Input: part model. Units: mm. Frame: model coordinates. A direction names the side the tool comes from. Give positions to 0.01 mm unless a question says otherwise; leave off trailing zeros. Loops run counter-clockwise (first coordinate to the right, second up) from the corner with the lowest first, then second, coordinate; pieces in that order, holes last. Notation, with made-up numbers: M 76,-25 L 90,-25 A24 cw 90,12 Z; hole C 22.25,50 d9. An arc over 180 degrees is marked long. Use CSV: the item, a comma, the result in double quotes. Start each with the question number.
Q1. Section A-A, the plane y = 227.5. Output: boundary loops of the cut face in (x, z), plus the area to 3 significant figures.
Q2. Pull-direction query (X, two-part tool) for faces 4 (the flat face through (-75, 186, 0)), 5 (the cylindrical face through (220, 0, 8)), 6 (the cylindrical face through (-249.76, 10.99, 7.4)); classes: released by +X, released by -X, zero draft, split by the parting line, or undercut.
Q3. Material intervals for line 1 along Y through (x, z) = (0, 8.75); line 2 along Y through (x, z) = (-113.75, 6.5); line 3 along Z through (x, y) = (199, -66), sorted ascending.
Q4. Section C-C, the plane z = -47. Output: boundary loops of the cut face in (x, y), plus the area to 3 significant figures.
Q5. Reachability of faces 1 (the cylindrical face through (117.211, 190.367, 7.605)), 2 (the cylindrical face through (187.903, -59.173, 3.99)), 3 (the cylindrical face through (-5.47, 24.65, -237.46)) from +Z, -Z, +X, -X, +Y, -Y: full face, straight path, thin tool, end or side. Return the list, or none.
Q6. Section B-B, the plane x = -112.5. State how many separate pieces and enclosed holes the cut face has, plus the area to 3 significant figures.
Q7. Pin query (flat end, axial travel): pin 1 (12 mm diameter, centred on y = 21.5, z = -73.5, fed in from +X); pin 2 (10 mm diameter, centred on y = 8, z = -139, fed in from -X); pin 3 (24 mm diameter, centred on x = 113.75, y = -197.02, fed in from -Z). Return the tip coordinate at first contact, or that it passes through.
from build123d import *

# Parameters (mm, degrees)
F0_R     = 250
F0_R_2   = 200
F1_DEPTH = 15
F4_R     = 7.5
F5_DEPTH = 15
F6_R     = 20
F7_DEPTH = 40
F8_R     = 25.25
F9_DEPTH = 5


with BuildPart() as f1:
    # F0 (on Top) → F1 (new body)
    with BuildSketch(Plane.XY):
        Circle(F0_R)
        Circle(F0_R_2, mode=Mode.SUBTRACT)
    extrude(amount=F1_DEPTH)

    # F2 (on Front) → F3 (revolve)
    with BuildSketch(Plane.XZ):
        with BuildLine():
            Line((200, -6.715729), (200, 15))
            Line((200, 15), (197, 15))
            Line((197, 15), (197, -6.715729))
            ThreePointArc((197, -6.715729), (195.705952, -13.221347), (192.020815, -18.736544))
            Line((192.020815, -18.736544), (18.757359, -192))
            Line((18.757359, -192), (0, -192))
            Line((0, -192), (0, -195))
            Line((0, -195), (20, -195))
            Line((20, -195), (194.142136, -20.857864))
            ThreePointArc((194.142136, -20.857864), (198.477591, -14.369397), (200, -6.715729))
        make_face()
    revolve(axis=Axis((0, 0, -193.5), (0, 0, -1)))

    # F4 (on face) → F5 (cut, through all)
    with BuildSketch(Plane.XY.offset(15)):
        with Locations((227.5, 0)):
            Circle(F4_R)
        with Locations((197.020779, 113.75)):
            Circle(F4_R)
        with Locations((113.75, 197.020779)):
            Circle(F4_R)
        with Locations((0, 227.5)):
            Circle(F4_R)
        with Locations((-113.75, 197.020779)):
            Circle(F4_R)
        with Locations((-197.020779, 113.75)):
            Circle(F4_R)
        with Locations((-227.5, 0)):
            Circle(F4_R)
        with Locations((-197.020779, -113.75)):
            Circle(F4_R)
        with Locations((-113.75, -197.020779)):
            Circle(F4_R)
        with Locations((0, -227.5)):
            Circle(F4_R)
        with Locations((113.75, -197.020779)):
            Circle(F4_R)
        with Locations((197.020779, -113.75)):
            Circle(F4_R)
    extrude(amount=-F5_DEPTH, mode=Mode.SUBTRACT)

    # F6 (on face) → F7 (join)
    with BuildSketch(Plane(origin=(0, 0, -195), x_dir=(1, 0, 0), z_dir=(0, 0, -1))):
        Circle(F6_R)
    extrude(amount=F7_DEPTH)

    # F8 (on face) → F9 (join)
    with BuildSketch(Plane(origin=(0, 0, -235), x_dir=(1, 0, 0), z_dir=(0, 0, -1))):
        Circle(F8_R)
    extrude(amount=F9_DEPTH)


solid = f1.part
A:
1,outline,"M -103.65,0 L -7.5,0 L -7.5,15 L -103.65,15 Z; M 7.5,0 L 103.65,0 L 103.65,15 L 7.5,15 Z"
1,area,"2,880 mm^2"
2,face 4,"zero draft"
2,face 5,"undercut"
2,face 6,"split by the parting line"
3,line 1,"-250 to -235, -220 to -197, 197 to 220, 235 to 250"
3,line 2,"-222.62 to -204.52, -189.52 to -160.84, 160.84 to 189.52, 204.52 to 222.62"
3,line 3,"0 to 15"
4,outline,"C 0,0 d336; hole C 0,0 d327.51"
4,area,"4,420 mm^2"
5,face 1,"+Z, -Z"
5,face 2,"+Z"
5,face 3,"-Z"
6,separate pieces,"3"
6,enclosed holes,"0"
6,area,"2,890 mm^2"
7,pin 1,"x = 145.99"
7,pin 2,"x = -80.63"
7,pin 3,"z = 0"
